Design review of the part shown in the three views and the two pictorial views. Dimensions are in mm from the part's minimum x, y and z. Coordinates: 2 decimals unless noted, no trailing zeros. Order: outer loops, then holes, each group sorted by start corner. A loop starts at its lowest first (then second) coordinate and runs counter-clockwise, first axis right, second up. Notation, with made-up numbers: (52.5, -1) -> (86.5, -1) arc R20 cw to (86.5, 22) -> close; hole circle Ø4 at (22, -20). An arc over 180 degrees is marked (long way). Answer as a JSON object with one key per item and string values. Group by question number.
1) Add section C-C, the plane z = 1.9. Write out the cut boundary in (x, y), then the cut area to 3 significant figures.
2) Draft analysis for pull direction X (two halves, no side actions). For the marked faces 1, 2 and 3, state which applies: +X half, -X half, draft (parallel to the pull), parting line (faces both ways), or undercut.
3) Wall thickness on L1, parallel to Y at x = 7, z = 2.15; L2, parallel to Y at x = 4, z = 1.2; L3, parallel to X at y = 9, z = 4.6: over which ranges is each line inside the solid? List them lowest first.
4) Add section A-A, the plane x = 7. Write out the cut boundary in (y, z), then the cut area to 4 significant figures.
5) For pin 1 (1 mm diameter, centred on x = 6, z = 4.5, fed in from -Y); pin 2 (3 mm diameter, centred on x = 6, z = 1.5, fed in from +Y); pin 3 (1 mm diameter, centred on x = 12, z = 0.5, fed in from +Y); pin 4 (1 mm diameter, centred on x = 9.5, y = 6, fed in from +Z), all flat-tipped, find the tip position at first contact; note any pin that passes through.
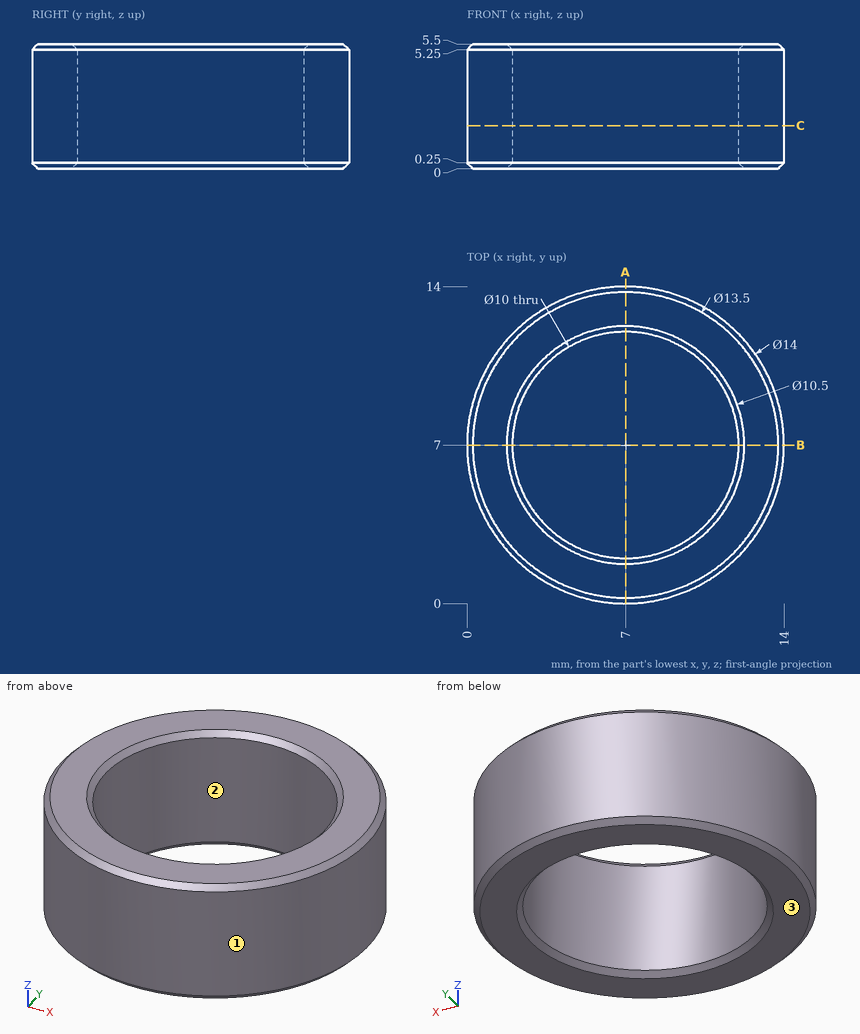
Output values:
{
 "1": {"outline": "circle Ø14 at (7, 7); hole circle Ø10 at (7, 7)", "area": "75.4 mm²"},
 "2": {"face 1": "parting line", "face 2": "undercut", "face 3": "draft"},
 "3": {"L1": "y = 0 to 2, 12 to 14", "L2": "y = 0.68 to 3, 11 to 13.32", "L3": "x = 0.29 to 2.42, 11.58 to 13.71"},
 "4": {"outline": "(0, 0.25) -> (0.25, 0) -> (1.75, 0) -> (2, 0.25) -> (2, 5.25) -> (1.75, 5.5) -> (0.25, 5.5) -> (0, 5.25) -> close; (12, 0.25) -> (12.25, 0) -> (13.75, 0) -> (14, 0.25) -> (14, 5.25) -> (13.75, 5.5) -> (12.25, 5.5) -> (12, 5.25) -> close", "area": "21.75 mm²"},
 "5": {"pin 1": "stops at y = 0.02", "pin 2": "stops at y = 14", "pin 3": "stops at y = 12.36", "pin 4": "passes through"}
}
